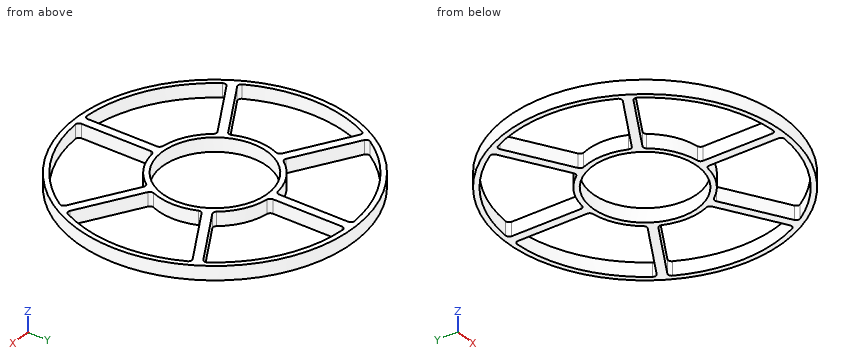
from build123d import *

# Parameters (mm, degrees)
SKETCH1_R           = 40
SKETCH1_R_2         = 15.2
BOSS_EXTRUDE1_DEPTH = 2
FILLET2_R           = 1


with BuildPart() as part:
    # Sketch1 → Boss-Extrude1 (new, symmetric)
    with BuildSketch(Plane.XY):
        Circle(SKETCH1_R)
        Circle(SKETCH1_R_2, mode=Mode.SUBTRACT)
        with BuildLine():
            ThreePointArc((1.25, -38.479702442), (19.25, -33.341978046), (32.699399845, -20.322382976))
            Line((32.699399845, -20.322382976), (13.797053425, -9.409108182))
            ThreePointArc((13.797053425, -9.409108182), (8.35, -14.462624243), (1.25, -16.653152855))
            Line((1.25, -16.653152855), (1.25, -38.479702442))
        make_face(mode=Mode.SUBTRACT)
        with BuildLine():
            ThreePointArc((33.949399845, -18.157319466), (38.5, 0), (33.949399845, 18.157319466))
            Line((33.949399845, 18.157319466), (15.047053425, 7.244044673))
            ThreePointArc((15.047053425, 7.244044673), (16.7, 0), (15.047053425, -7.244044673))
            Line((15.047053425, -7.244044673), (33.949399845, -18.157319466))
        make_face(mode=Mode.SUBTRACT)
        with BuildLine():
            ThreePointArc((-1.25, 38.479702442), (-19.25, 33.341978046), (-32.699399845, 20.322382976))
            Line((-32.699399845, 20.322382976), (-13.797053425, 9.409108182))
            ThreePointArc((-13.797053425, 9.409108182), (-8.35, 14.462624243), (-1.25, 16.653152855))
            Line((-1.25, 16.653152855), (-1.25, 38.479702442))
        make_face(mode=Mode.SUBTRACT)
        with BuildLine():
            ThreePointArc((-32.699399845, -20.322382976), (-19.25, -33.341978046), (-1.25, -38.479702442))
            Line((-1.25, -38.479702442), (-1.25, -16.653152855))
            ThreePointArc((-1.25, -16.653152855), (-8.35, -14.462624243), (-13.797053425, -9.409108182))
            Line((-13.797053425, -9.409108182), (-32.699399845, -20.322382976))
        make_face(mode=Mode.SUBTRACT)
        with BuildLine():
            Line((-15.047053425, 7.244044673), (-33.949399845, 18.157319466))
            ThreePointArc((-33.949399845, 18.157319466), (-38.5, 0), (-33.949399845, -18.157319466))
            Line((-33.949399845, -18.157319466), (-15.047053425, -7.244044673))
            ThreePointArc((-15.047053425, -7.244044673), (-16.7, 0), (-15.047053425, 7.244044673))
        make_face(mode=Mode.SUBTRACT)
        with BuildLine():
            Line((13.797053425, 9.409108182), (32.699399845, 20.322382976))
            ThreePointArc((32.699399845, 20.322382976), (19.25, 33.341978046), (1.25, 38.479702442))
            Line((1.25, 38.479702442), (1.25, 16.653152855))
            ThreePointArc((1.25, 16.653152855), (8.35, 14.462624243), (13.797053425, 9.409108182))
        make_face(mode=Mode.SUBTRACT)
    extrude(amount=BOSS_EXTRUDE1_DEPTH, both=True)

    # Fillet2
    fillet2_edges = [part.edges().sort_by_distance(p)[0] for p in [
        (32.699399845, 20.322382976, 0),
        (1.25, 38.479702442, 0),
        (1.25, 16.653152855, 0),
        (13.797053425, 9.409108182, 0),
        (-33.949399845, 18.157319466, 0),
        (-33.949399845, -18.157319466, 0),
        (-15.047053425, -7.244044673, 0),
        (-15.047053425, 7.244044673, 0),
        (-1.25, -38.479702442, 0),
        (-1.25, -16.653152855, 0),
        (-13.797053425, -9.409108182, 0),
        (-32.699399845, -20.322382976, 0),
        (-32.699399845, 20.322382976, 0),
        (-13.797053425, 9.409108182, 0),
        (-1.25, 16.653152855, 0),
        (-1.25, 38.479702442, 0),
        (33.949399845, 18.157319466, 0),
        (15.047053425, 7.244044673, 0),
        (15.047053425, -7.244044673, 0),
        (33.949399845, -18.157319466, 0),
        (32.699399845, -20.322382976, 0),
        (13.797053425, -9.409108182, 0),
        (1.25, -16.653152855, 0),
        (1.25, -38.479702442, 0),
    ]]
    fillet(fillet2_edges, radius=FILLET2_R)


solid = part.part
Read the model definition and answer for the solid it produces. Units are mm, in the model's axes. Round coordinates to 2 decimals unless told otherwise and drop trailing zeros. Order: outer loops, then holes, each group sorted by start corner. A loop starts at its lowest first (then second) coordinate and runs counter-clockwise, first axis right, second up.
1) Flat-ended cylindrical pins translate along their axes: pin 1 (2 mm diameter, centred on y = -28.5, z = 1, fed in from +X); pin 2 (2 mm diameter, centred on y = 25, z = -1, fed in from +X); pin 3 (2 mm diameter, centred on y = -6.5, z = 1.5, fed in from -X); pin 4 (18 mm diameter, centred on x = 0, y = 0, fed in from -Z). Find the tip coordinate at first contact, or state that the pin passes through.
2) Straight lines are drawn through the part: L1, parallel to X at y = 20.5, z = 0.4; L2, parallel to X at y = 23, z = 1.55; L3, parallel to X at y = -14, z = 0.1. For each, find the intervals that lie inside material, in ascending order.
3) The part is cut by section D-D on y = -27.5. Write down the section's boundary in (x, z), plus the area to 3 significant figures.
4) The part is cut by section B-B on y = 0. Write down the section's boundary in (x, z), plus the area to 3 significant figures.
5) The part is cut by section A-A on x = 0. Write down the section's boundary in (y, z), plus the area to 3 significant figures.
6) The part is cut by section C-C on x = -26. Write down the section's boundary in (y, z).
Resolved:
1. pin 1: stops at x = 29.05
1. pin 2: stops at x = 32
1. pin 3: stops at x = -39.62
1. pin 4: passes through
2. L1: x = -34.35 to -32.28, -1.25 to 1.25, 32.28 to 34.35
2. L2: x = -32.73 to -30.87, -1.25 to 1.25, 30.87 to 32.73
2. L3: x = -37.47 to -35.86, -26.75 to -21.75, -9.1 to -5.92, 5.92 to 9.1, 21.75 to 26.75, 35.86 to 37.47
3. outline: (-29.05, -2) - (-26.94, -2) - (-26.94, 2) - (-29.05, 2) - close; (-1.25, -2) - (1.25, -2) - (1.25, 2) - (-1.25, 2) - close; (26.94, -2) - (29.05, -2) - (29.05, 2) - (26.94, 2) - close
3. area: 26.8 mm2
4. outline: (-40, -2) - (-38.5, -2) - (-38.5, 2) - (-40, 2) - close; (-16.7, -2) - (-15.2, -2) - (-15.2, 2) - (-16.7, 2) - close; (15.2, -2) - (16.7, -2) - (16.7, 2) - (15.2, 2) - close; (38.5, -2) - (40, -2) - (40, 2) - (38.5, 2) - close
4. area: 24.0 mm2
5. outline: (-40, -2) - (-15.2, -2) - (-15.2, 2) - (-40, 2) - close; (15.2, -2) - (40, -2) - (40, 2) - (15.2, 2) - close
5. area: 198 mm2
6. outline: (-30.4, -2) - (-28.39, -2) - (-28.39, 2) - (-30.4, 2) - close; (-16.45, -2) - (-13.57, -2) - (-13.57, 2) - (-16.45, 2) - close; (13.57, -2) - (16.45, -2) - (16.45, 2) - (13.57, 2) - close; (28.39, -2) - (30.4, -2) - (30.4, 2) - (28.39, 2) - close
